Geometry: final body of the model. Coordinates: model frame, mm. Round coordinates to 2 decimals unless told otherwise and drop trailing zeros. Loops run counter-clockwise (first coordinate to the right, second up) from the corner with the lowest first, then second, coordinate; pieces in that order, holes last. Notation, with made-up numbers: (65.25, -16) -> (96.25, -16) arc R19 ccw to (96.25, -12) -> close; hole circle Ø8 at (34, 4.5). An arc over 180 degrees is marked (long way). Answer in a Markdown table with one row per item.
```python
from build123d import *

# Parameters (mm, degrees)
SKETCH_1_W      = 25
SKETCH_1_H      = 5
EXTRUDE_1_DEPTH = 5.5
FILLET_1_R      = 100


with BuildPart() as part:
    # 草图1 → 凸台-拉伸1 (new body)
    with BuildSketch(Plane.XY):
        Polygon((-15, 20), (-65, 16), (-115, 20), (-130, 20), (-130, 0), (-117.5, 0), (-117.5, 6), (-119, 6), (-119, 8.9), (-117.5, 8.9), (-117.5, 11), (-113.5, 11), (-113.5, 8.9), (-112, 8.9), (-112, 6), (-113.5, 6), (-113.5, 0), (-108, 0), (-108, -5), (-93, -5), (-93, 0), (-37, 0), (-37, -5), (-22, -5), (-22, 0), (-16.5, 0), (-16.5, 6), (-18, 6), (-18, 8.9), (-16.5, 8.9), (-16.5, 11), (-12.5, 11), (-12.5, 8.9), (-11, 8.9), (-11, 6), (-12.5, 6), (-12.5, 0), (0, 0), (0, 20), align=None)
        with Locations((-65, 10.5)):
            Rectangle(SKETCH_1_W, SKETCH_1_H, mode=Mode.SUBTRACT)
    extrude(amount=EXTRUDE_1_DEPTH)

    # 圆角1
    fillet_1_edges = [part.edges().sort_by_distance(p)[0] for p in [
        (-65, 16, 2.75),
    ]]
    fillet(fillet_1_edges, radius=FILLET_1_R)


solid = part.part
```
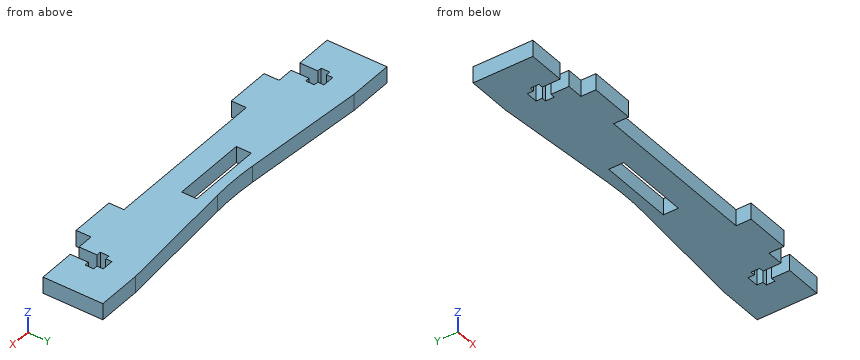
Item 1: Section query A-A, the plane x = -59.5. Output: boundary loops of the cut face in (y, z), and give its area (3 significant figures).
Ans:
| item | result |
|---|---|
| outline | (0, 0) -> (8, 0) -> (8, 5.5) -> (0, 5.5) -> close; (13, 0) -> (16.47, 0) -> (16.47, 5.5) -> (13, 5.5) -> close |
| area | 63.1 mm2 |
Item 2: Ray query, L1, parallel to X at y = 2.75, z = 1.75; L2, parallel to X at y = 8.25, z = 4.45; L3, parallel to X at y = 7, z = 3.35. Return the intervals inside material, ascending.
Ans:
| item | result |
|---|---|
| L1 | -130 to -117.5, -113.5 to -16.5, -12.5 to 0 |
| L2 | -130 to -119, -112 to -77.5, -52.5 to -18, -11 to 0 |
| L3 | -130 to -119, -112 to -18, -11 to 0 |
Item 3: First-contact query: P1, Ø3, axis at x = -69.5, z = 2.5, coming from the +Y side; P2, Ø1.2, axis at x = -15, z = 2, coming from the -Y side; P3, Ø1.6, axis at x = -3.5, z = 3.5, coming from the -Y side. Flat tips, straight axial feed; report the tip coordinate or a pass-through.
Ans:
| item | result |
|---|---|
| P1 | y = 16.5 |
| P2 | y = 11 |
| P3 | y = 0 |
Item 4: Section query C-C, the plane x = -46. Output: boundary loops of the cut face in (y, z).
Ans:
| item | result |
|---|---|
| outline | (0, 0) -> (17.52, 0) -> (17.52, 5.5) -> (0, 5.5) -> close |
Item 5: Section query D-D, the plane x = -8.5. Output: boundary loops of the cut face in (y, z), and give its area (3 significant figures).
Ans:
| item | result |
|---|---|
| outline | (0, 0) -> (20, 0) -> (20, 5.5) -> (0, 5.5) -> close |
| area | 110 mm2 |
Item 6: Section query B-B, the plane y = 17.75. Output: boundary loops of the cut face in (x, z) (3 decimals).
Ans:
| item | result |
|---|---|
| outline | (-130, 0) -> (-86.875, 0) -> (-86.875, 5.5) -> (-130, 5.5) -> close; (-43.125, 0) -> (0, 0) -> (0, 5.5) -> (-43.125, 5.5) -> close |
